from build123d import *

# Parameters (mm, degrees)
SKETCH_1_W          = 35.2
SKETCH_1_H          = 43
EXTRUDE_1_DEPTH     = 4
SKETCH_2_W          = 35.2
SKETCH_2_H          = 25
EXTRUDE_2_DEPTH     = 32
SKETCH_4_R          = 12.5
CUT_EXTRUDE_1_DEPTH = 32
SKETCH_6_R          = 2
CUT_EXTRUDE_2_DEPTH = 32
SKETCH_7_W          = 35.2
SKETCH_7_H          = 36
EXTRUDE_3_DEPTH     = 3
SKETCH_8_R          = 3.5
SKETCH_8_R_2        = 1.5
CUT_EXTRUDE_3_DEPTH = 10


with BuildPart() as part:
    # Эскиз1 → Бобышка-Вытянуть1 (new body)
    with BuildSketch(Plane.XY):
        Rectangle(SKETCH_1_W, SKETCH_1_H)
    extrude(amount=EXTRUDE_1_DEPTH)

    # Эскиз2 → Бобышка-Вытянуть2 (add)
    with BuildSketch(Plane.XY.offset(4)):
        with Locations((0, 9)):
            Rectangle(SKETCH_2_W, SKETCH_2_H)
    extrude(amount=EXTRUDE_2_DEPTH)

    # Эскиз4 → Вырез-Вытянуть1 (cut)
    with BuildSketch(Plane.XZ.offset(3.5)):
        with Locations(Location((0, 20, 0), (0, 0, 270))):
            Circle(SKETCH_4_R)
    extrude(amount=-CUT_EXTRUDE_1_DEPTH, mode=Mode.SUBTRACT)

    # Эскиз6 → Вырез-Вытянуть2 (cut)
    with BuildSketch(Plane.XY.offset(4)):
        with Locations((0, -7.5)):
            Circle(SKETCH_6_R)
        with Locations((0, -17.5)):
            Circle(SKETCH_6_R)
    extrude(amount=-CUT_EXTRUDE_2_DEPTH, mode=Mode.SUBTRACT)

    # Эскиз7 → Бобышка-Вытянуть3 (add)
    with BuildSketch(Plane(origin=(0, 21.5, 0), x_dir=(1, 0, 0), z_dir=(0, 1, 0))):
        with Locations((0, -18)):
            Rectangle(SKETCH_7_W, SKETCH_7_H)
    extrude(amount=EXTRUDE_3_DEPTH)

    # Эскиз8 → Вырез-Вытянуть3 (cut)
    with BuildSketch(Plane(origin=(0, 24.5, 0), x_dir=(1, 0, 0), z_dir=(0, 1, 0))):
        with Locations(Location((0, -20, 0), (0, 0, 270))):
            Circle(SKETCH_8_R)
        with Locations(Location((8.4, -20, 0), (0, 0, 270))):
            Circle(SKETCH_8_R_2)
        with Locations(Location((-8.4, -20, 0), (0, 0, 270))):
            Circle(SKETCH_8_R_2)
    extrude(amount=-CUT_EXTRUDE_3_DEPTH, mode=Mode.SUBTRACT)


solid = part.part
Input: part model. Units: mm. Frame: model coordinates. A direction names the side the tool comes from. Give positions to 0.01 mm unless a question says otherwise; leave off trailing zeros. Loops run counter-clockwise (first coordinate to the right, second up) from the corner with the lowest first, then second, coordinate; pieces in that order, holes last. Notation, with made-up numbers: (74.25, 32) -> (114.25, 32) arc R23 ccw to (114.25, 51) -> close; hole circle Ø9 at (-29.75, 74). An arc over 180 degrees is marked (long way). Answer as a JSON object with one key per item and string values. Group by question number.
Item 1: Cut plane A-A, the plane y = -17.5. Return the cut outline in (x, z).
Item 2: Cut plane C-C, the plane x = 0. Return the cut outline in (y, z).
Item 3: Line query: probe 1 along X at (y, z) = (23.75, 20); probe 2 along X at (y, z) = (3, 20); probe 3 along Y at (x, z) = (-3.5, 24). Output: solid intervals per line, ascending.
Item 4: Cut plane B-B, the plane z = 20. Return the cut outline in (x, y), and give its area (3 significant figures).
Item 5: Pull-direction query (Z, two-part tool) for faces 4 (the flat face through (0, -12, 4)), 5 (the cylindrical face through (-8.33, 23.02, 18.5)), 6 (the flat face through (-17.6, 11, 18)); classes: released by +Z, released by -Z, zero draft, split by the parting line, or undercut.
Item 6: Cut plane D-D, the plane x = -8.4. Return the cut outline in (y, z), and give its area (3 significant figures).
Item 7: Reachability of faces 1 (the flat face through (-8, -3.5, 9)), 2 (the flat face through (17.6, 11, 18)), 3 (the cylindrical face through (8.45, 8.82, 29.21)) from +Z, -Z, +X, -X, +Y, -Y: full face, straight path, thin tool, end or side. Return the list, or none.
Item 8: Pin query (flat end, axial travel): P1, Ø5.5, axis at x = 7.5, y = -16.5, coming from the +Z side; P2, Ø8, axis at x = 0, z = 20, coming from the -Y side. Return the tip coordinate at first contact, or that it passes through.
Checks:
{
 "1": {"outline": "(-17.6, 0) -> (-2, 0) -> (-2, 4) -> (-17.6, 4) -> close; (2, 0) -> (17.6, 0) -> (17.6, 4) -> (2, 4) -> close"},
 "2": {"outline": "(-21.5, 0) -> (-19.5, 0) -> (-19.5, 4) -> (-21.5, 4) -> close; (-15.5, 0) -> (-9.5, 0) -> (-9.5, 4) -> (-15.5, 4) -> close; (-5.5, 0) -> (24.5, 0) -> (24.5, 16.5) -> (21.5, 16.5) -> (21.5, 7.5) -> (-3.5, 7.5) -> (-3.5, 4) -> (-5.5, 4) -> close; (-3.5, 32.5) -> (21.5, 32.5) -> (21.5, 23.5) -> (24.5, 23.5) -> (24.5, 36) -> (-3.5, 36) -> close"},
 "3": {"probe 1": "x = -17.6 to -9.9, -6.9 to -3.5, 3.5 to 6.9, 9.9 to 17.6", "probe 2": "x = -17.6 to -12.5, 12.5 to 17.6", "probe 3": "y = 21.5 to 24.5"},
 "4": {"outline": "(-17.6, -3.5) -> (-12.5, -3.5) -> (-12.5, 21.5) -> (-9.9, 21.5) -> (-9.9, 24.5) -> (-17.6, 24.5) -> close; (-6.9, 21.5) -> (-3.5, 21.5) -> (-3.5, 24.5) -> (-6.9, 24.5) -> close; (3.5, 21.5) -> (6.9, 21.5) -> (6.9, 24.5) -> (3.5, 24.5) -> close; (9.9, 21.5) -> (12.5, 21.5) -> (12.5, -3.5) -> (17.6, -3.5) -> (17.6, 24.5) -> (9.9, 24.5) -> close", "area": "322 mm²"},
 "5": {"face 4": "released by +Z", "face 5": "undercut", "face 6": "zero draft"},
 "6": {"outline": "(-21.5, 0) -> (24.5, 0) -> (24.5, 18.5) -> (21.5, 18.5) -> (21.5, 10.74) -> (-3.5, 10.74) -> (-3.5, 4) -> (-21.5, 4) -> close; (-3.5, 29.26) -> (21.5, 29.26) -> (21.5, 21.5) -> (24.5, 21.5) -> (24.5, 36) -> (-3.5, 36) -> close", "area": "608 mm²"},
 "7": {"face 1": "+Z, +X, -X, -Y", "face 2": "+Z, -Z, +X, +Y, -Y", "face 3": "-Y"},
 "8": {"P1": "stops at z = 4", "P2": "stops at y = 21.5"}
}
